```python
from build123d import *

# Parameters (mm, degrees)
SKETCH_1_R          = 7
SKETCH_1_R_2        = 1.25
EXTRUDE_1_DEPTH     = 7.5
SKETCH_2_R          = 1.3
CUT_EXTRUDE_1_DEPTH = 7.5
CHAMFER_1_SIZE      = 0.2


with BuildPart() as part:
    # Sketch 1 → Extrude 1 (new body)
    with BuildSketch(Plane.XY):
        with BuildLine():
            Line((0, -33), (-30, -33))
            Line((-30, -33), (-16.529573398, 5.746581877))
            ThreePointArc((-16.529573398, 5.746581877), (0, 17.5), (16.529573398, 5.746581877))
            Line((16.529573398, 5.746581877), (30, -33))
            Line((30, -33), (0, -33))
        make_face()
        Circle(SKETCH_1_R, mode=Mode.SUBTRACT)
        with Locations((-6, 12)):
            Circle(SKETCH_1_R_2, mode=Mode.SUBTRACT)
        with Locations((-12, 6)):
            Circle(SKETCH_1_R_2, mode=Mode.SUBTRACT)
        with Locations((-12, -6)):
            Circle(SKETCH_1_R_2, mode=Mode.SUBTRACT)
        with Locations((6, 12)):
            Circle(SKETCH_1_R_2, mode=Mode.SUBTRACT)
        with Locations((12, 6)):
            Circle(SKETCH_1_R_2, mode=Mode.SUBTRACT)
        with Locations((12, -6)):
            Circle(SKETCH_1_R_2, mode=Mode.SUBTRACT)
    extrude(amount=-EXTRUDE_1_DEPTH)

    # Sketch 2 → Cut-Extrude 1 (cut)
    with BuildSketch(Plane(origin=(0, -33, 0), x_dir=(-1, 0, 0), z_dir=(0, -1, 0))):
        with Locations(Location((-18, 3.75, 0), (0, 0, 180))):
            Circle(SKETCH_2_R)
        with Locations(Location((-6, 3.75, 0), (0, 0, 180))):
            Circle(SKETCH_2_R)
        with Locations(Location((6, 3.75, 0), (0, 0, 180))):
            Circle(SKETCH_2_R)
        with Locations(Location((18, 3.75, 0), (0, 0, 180))):
            Circle(SKETCH_2_R)
    extrude(amount=-CUT_EXTRUDE_1_DEPTH, mode=Mode.SUBTRACT)

    # Chamfer 1
    chamfer_1_edges = [part.edges().sort_by_distance(p)[0] for p in [
        (16.7, -33, -3.75),
        (4.7, -33, -3.75),
        (-7.3, -33, -3.75),
        (-19.3, -33, -3.75),
    ]]
    chamfer(chamfer_1_edges, length=CHAMFER_1_SIZE)


solid = part.part
```
Geometry check sheet. Reference: the model listing, model coordinates, mm. A direction names the side the tool comes from. Round coordinates to 2 decimals unless told otherwise and drop trailing zeros. Write each loop counter-clockwise with the first axis right and the second up, starting at its lowest first coordinate (ties: lowest second). Pieces come first, ordered by that corner, then holes. Notation, with made-up numbers: (68.5, 1.25) -> (124.5, 1.25) arc R8 cw to (124.5, 10.25) -> close; hole circle Ø6 at (72, 61.25). An arc over 180 degrees is marked (long way). Put each result on its own line as item: value.
1) Cross-section at B-B, the plane x = -12. Enter the section's corners in (y, z), plus the area to 3 significant figures.
Recorded:
outline: (-33, -7.5) -> (-7.25, -7.5) -> (-7.25, 0) -> (-33, 0) -> close; (-4.75, -7.5) -> (4.75, -7.5) -> (4.75, 0) -> (-4.75, 0) -> close; (7.25, -7.5) -> (12.74, -7.5) -> (12.74, 0) -> (7.25, 0) -> close
area: 306 mm2
2) Access from +Z, -Z, +X, -X, +Y, -Y to the whole of each face (thin tool, end or side, straight path). Record for faces 5 (the face through (-0.303, 17.497, -3.698)), 6 (the face through (7.24, -29.2, -3.36)).
Recorded:
face 5: +Z, -Z, +Y
face 6: -Y
3) Depth check by flat-ended pin: P1, Ø3, axis at x = 12, y = -6, coming from the +Z side; P2, Ø3, axis at x = -9.5, z = -3.5, coming from the +Y side; P3, Ø3, axis at y = -4, z = -1, coming from the +X side; P4, Ø1, axis at y = -15.5, z = -3, coming from the -X side. Enter the tip coordinate at first touch or a pass-through.
Recorded:
P1: stops at z = 0
P2: stops at y = 15.56
P3: stops at x = 20.44
P4: stops at x = -24.09
4) Release check for a two-part mould opening along Y. For faces 1 (the face through (-19.3, -29.2, -3.7)), 2 (the face through (11.73, -7.22, -3.7)), 3 (the face through (-6.16, 13.24, -3.7)), 4 (the face through (6, -25.5, -4)) record: pulls with the +Y half, pulls with the -Y half, needs draft (parallel to the pull), parting line crosses it, or undercut.
Recorded:
face 1: needs draft
face 2: undercut
face 3: undercut
face 4: pulls with the -Y half
5) Cross-section at C-C, the plane y = 12. Enter the section's corners in (x, z).
Recorded:
outline: (-12.74, -7.5) -> (-7.25, -7.5) -> (-7.25, 0) -> (-12.74, 0) -> close; (-4.75, -7.5) -> (4.75, -7.5) -> (4.75, 0) -> (-4.75, 0) -> close; (7.25, -7.5) -> (12.74, -7.5) -> (12.74, 0) -> (7.25, 0) -> close
6) Cross-section at A-A, the plane z = -6. Enter the section's corners in (x, y).
Recorded:
outline: (-30, -33) -> (30, -33) -> (16.53, 5.75) arc R17.5 ccw to (-16.53, 5.75) -> close; hole circle Ø2.5 at (-12, -6); hole circle Ø2.5 at (-12, 6); hole circle Ø2.5 at (-6, 12); hole circle Ø14 at (0, 0); hole circle Ø2.5 at (6, 12); hole circle Ø2.5 at (12, -6); hole circle Ø2.5 at (12, 6)
7) Thickness scan on probe 1 along Y at (x, z) = (0, -4.5); probe 2 along Z at (x, y) = (-6, -29); probe 3 along Y at (x, z) = (-6, -3.25). Record the ranges inside material, lowest first. Write a range as from..to.
Recorded:
probe 1: y = -33..-7, 7..17.5
probe 2: z = -7.5..-5.05, -2.45..0
probe 3: y = -25.5..-3.61, 3.61..10.75, 13.25..16.44
8) Cross-section at D-D, the plane y = 3.5. Enter the section's corners in (x, z), plus the area to 3 significant figures.
Recorded:
outline: (-17.31, -7.5) -> (-6.06, -7.5) -> (-6.06, 0) -> (-17.31, 0) -> close; (6.06, -7.5) -> (17.31, -7.5) -> (17.31, 0) -> (6.06, 0) -> close
area: 169 mm2
